CAD build for the part. Positions are in the model's coordinates, mm. Round coordinates to 2 decimals unless told otherwise and drop trailing zeros. Loops run counter-clockwise (first coordinate to the right, second up) from the corner with the lowest first, then second, coordinate; pieces in that order, holes last.
```python
from build123d import *

# Parameters (mm, degrees)
F1_DEPTH = 20
F2_W     = 76.2
F2_H     = 76.2
F3_DEPTH = 40
F4_W     = 19.9898
F4_H     = 41.2496
F5_DEPTH = 20
F7_DEPTH = 251.162639


with BuildPart() as f1:
    # F0 (on Front) → F1 (new body)
    with BuildSketch(Plane.XZ):
        Polygon((121.926413, 229.678165), (-154.984387, 229.678165), (-258.438587, 50.490234), (-258.438587, -52.166674), (-154.984387, -231.354605), (121.926413, -231.354605), (225.380613, -52.166674), (225.380613, 50.490234), align=None)
    extrude(amount=F1_DEPTH)

    # F2 (on face) → F3 (join)
    with BuildSketch(Plane(origin=(0, 0, 0), x_dir=(-1, 0, 0), z_dir=(0, 1, 0))):
        with Locations((-187.280613, -0.817766)):
            Rectangle(F2_W, F2_H)
    extrude(amount=F3_DEPTH)

    # F4 (on face) → F5 (join)
    with BuildSketch(Plane.YZ.offset(225.380613)):
        with Locations((19.9009, -0.817766)):
            Rectangle(F4_W, F4_H)
    extrude(amount=F5_DEPTH)

    # F6 (on face) → F7 (cut, through all)
    with BuildSketch(Plane.XY.offset(19.807034)):
        Polygon((245.380613, 29.8958), (225.380613, 29.8958), (245.380613, 9.906), align=None)
    extrude(amount=-F7_DEPTH, mode=Mode.SUBTRACT)


solid = f1.part
```
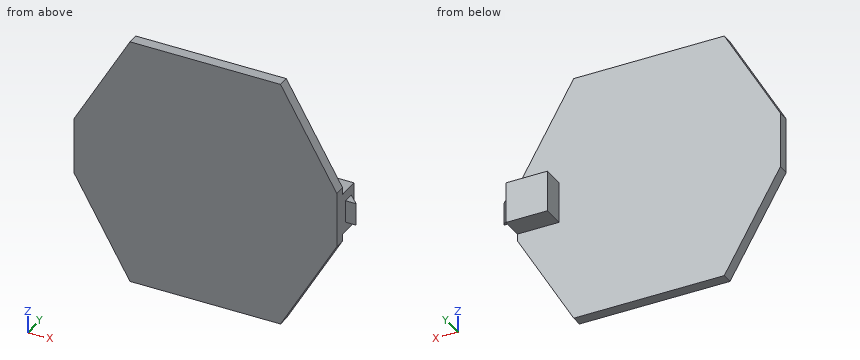
Item 1: Cut at D-D, the plane x = -83. Give the cut face in (y, z), plus the area to 3 significant figures.
Answers follow:
outline: (-20, -231.35) - (0, -231.35) - (0, 229.68) - (-20, 229.68) - close
area: 9,220 mm2
Item 2: Cut at B-B, the plane x = 163. Give the cut face in (y, z).
Answers follow:
outline: (-20, -160.21) - (0, -160.21) - (0, -38.92) - (40, -38.92) - (40, 37.28) - (0, 37.28) - (0, 158.54) - (-20, 158.54) - close
Item 3: Cut at C-C, the plane z = 85. Give the cut face in (x, y), plus the area to 3 significant figures.
Answers follow:
outline: (-238.51, -20) - (205.46, -20) - (205.46, 0) - (-238.51, 0) - close
area: 8,880 mm2
Item 4: Probe line 1 (Y direction, x = 141.5, z = 167); line 2 (Z direction, x = 181, y = 9); line 3 (X direction, y = -2, z = -115). List the from-to ranges inside material, lowest first.
Answers follow:
line 1: y = -20 to 0
line 2: z = -38.92 to 37.28
line 3: x = -222.16 to 189.1
Item 5: Cut at A-A, the plane y = -13. Give the cut face in (x, z).
Answers follow:
outline: (-258.44, -52.17) - (-154.98, -231.35) - (121.93, -231.35) - (225.38, -52.17) - (225.38, 50.49) - (121.93, 229.68) - (-154.98, 229.68) - (-258.44, 50.49) - close
Item 6: Flat gauge pins, fed straight in: P1, Ø12, axis at x = 179.5, y = 25, coming from the +Z side; P2, Ø22, axis at x = 239, z = -6.5, coming from the -Y side; P3, Ø22, axis at x = 239.5, y = 18.5, coming from the -Z side. Where does each tip first touch, or does it go through?
Answers follow:
P1: stops at z = 37.28
P2: stops at y = 9.91
P3: stops at z = -21.44
